```python
from build123d import *

# Parameters (mm, degrees)
F1_DEPTH       = 5
F2_W           = 19.9294948324
F2_H           = 5
F3_DEPTH       = 20
F5_D           = 6.8
F7_D           = 3.2
F7_CSINK_D     = 6.72
F7_CSINK_ANGLE = 90


with BuildPart() as f1:
    # F0 (on Front) → F1 (new body)
    with BuildSketch(Plane.XZ):
        with BuildLine():
            Line((9.9294948324, -23), (9.9294948324, -1.1853827958))
            ThreePointArc((9.9294948324, -1.1853827958), (0.5937388633, 9.9823581464), (-10, 0))
            Line((-10, 0), (-10, -23))
            Line((-10, -23), (9.9294948324, -23))
        make_face()
    extrude(amount=F1_DEPTH)

    # F2 (on face) → F3 (join)
    with BuildSketch(Plane.XZ.offset(5)):
        with Locations((-0.0352525838, -20.5)):
            Rectangle(F2_W, F2_H)
    extrude(amount=F3_DEPTH)

    # F5 (through all)
    with Locations(Plane(origin=(0, 0, 0), x_dir=(-1, 0, 0), z_dir=(0, 1, 0))):
        with Locations((0, 0)):
            Hole(F5_D / 2)

    # F7 (through all)
    with Locations(Plane.XY.offset(-18)):
        with Locations((0, -15)):
            CounterSinkHole(F7_D / 2, F7_CSINK_D / 2, counter_sink_angle=F7_CSINK_ANGLE)


solid = f1.part
```
Input: part model. Units: mm. Frame: model coordinates. A direction names the side the tool comes from. Give positions to 0.01 mm unless a question says otherwise; leave off trailing zeros. Order: outer loops, then holes, each group sorted by start corner. A loop starts at its lowest first (then second) coordinate and runs counter-clockwise, first axis right, second up. Notation, with made-up numbers: M 43.25,29 L 83.25,29 A25 cw 83.25,46 Z; hole C -25,59.5 d1. An arc over 180 degrees is marked long. Return JSON: item names as keys, results as strings.
1) Line query: L1, parallel to Z at x = 0, y = -1.3; L2, parallel to X at y = -15, z = -20.5; L3, parallel to Y at x = 0, z = -20.75. Output: solid intervals per line, ascending. Write a range as [from, to].
Taken from the geometry:
{"L1": "z = [-23, -3.4], [3.4, 10]", "L2": "x = [-10, -1.6], [1.6, 9.93]", "L3": "y = [-25, -16.6], [-13.4, 0]"}
2) Access query for faces 5 (the face through (-5, -15, -18)), 6 (the face through (0, -12, -23)). Directions: +Z, -Z, +X, -X, +Y, -Y. A direction counts if a zero-diameter tool reaches every point of the face in a straight line with its end or side. Return the directions, or none.
Taken from the geometry:
{"face 5": "+Z, +X, -X, -Y", "face 6": "-Z, +X, -X, +Y, -Y"}
3) Section query C-C on z = -5. Output: boundary loops of the cut face in (x, y), and give its area (3 significant figures).
Taken from the geometry:
{"outline": "M -10,-5 L 9.93,-5 L 9.93,0 L -10,0 Z", "area": "99.6 mm2"}
4) Section query A-A on y = -15. Output: boundary loops of the cut face in (x, z), and give its area (4 significant figures).
Taken from the geometry:
{"outline": "M -10,-23 L -1.6,-23 L -1.6,-19.76 L -3.36,-18 L -10,-18 Z; M 1.6,-23 L 9.93,-23 L 9.93,-18 L 3.36,-18 L 1.6,-19.76 Z", "area": "80.55 mm2"}
5) Section query B-B on x = 0. Output: boundary loops of the cut face in (y, z).
Taken from the geometry:
{"outline": "M -25,-23 L -16.6,-23 L -16.6,-19.76 L -18.36,-18 L -25,-18 Z; M -13.4,-23 L 0,-23 L 0,-3.4 L -5,-3.4 L -5,-18 L -11.64,-18 L -13.4,-19.76 Z; M -5,3.4 L 0,3.4 L 0,10 L -5,10 Z"}
6) Mould query, pull axis Y, two halves, no side actions, for faces 1 (the face through (0, -5, -4)), 2 (the face through (9.929, -7, -20)), 3 (the face through (0.208, -13.414, -21.403)), 4 (the face through (0, 0, -6)). Classes: released by +Y, released by -Y, zero draft, split by the parting line, or undercut.
Taken from the geometry:
{"face 1": "released by -Y", "face 2": "zero draft", "face 3": "undercut", "face 4": "released by +Y"}
7) Contact query for flat-ended pins moving along their axis: pin 1 (6 mm diameter, centred on x = 2.5, y = -15, fed in from +Z); pin 2 (4 mm diameter, centred on x = -4, z = -16.5, fed in from +Y); pin 3 (9 mm diameter, centred on x = 0, z = 0, fed in from -Y); pin 4 (1.9 mm diameter, centred on x = 0, y = -15, fed in from +Z). Output: stop coordinate, or through.
Taken from the geometry:
{"pin 1": "stops at z = -18", "pin 2": "stops at y = 0", "pin 3": "stops at y = -5", "pin 4": "passes through"}
8) Section query D-D on y = -9.5. Output: boundary loops of the cut face in (x, z).
Taken from the geometry:
{"outline": "M -10,-23 L 9.93,-23 L 9.93,-18 L -10,-18 Z"}
